Design review of the part built by this model. Coordinates are the model's own, in mm. Give positions to 0.01 mm unless a question says otherwise; leave off trailing zeros. Write each loop counter-clockwise with the first axis right and the second up, starting at its lowest first coordinate (ties: lowest second). Pieces come first, ordered by that corner, then holes. Notation, with made-up numbers: (1, -30.5) -> (25, -30.5) arc R36 ccw to (25, 8.5) -> close; hole circle Ø2 at (-30.5, -14.5). An arc over 180 degrees is marked (long way). Answer as a JSON object with one key per item and string values.
```python
from build123d import *

# Parameters (mm, degrees)
BOSS_EXTRU_1_DEPTH           = 1.6
BOSS_EXTRU_2_DEPTH           = 1.6
R_P_TITION_CIRCULAIRE1_COUNT = 24


with BuildPart() as part:
    # Esquisse1 → Boss.-Extru.1 (new body)
    with BuildSketch(Plane(origin=(0, 0, 0), x_dir=(1, 0, 0), z_dir=(0, 1, 0))):
        with BuildLine():
            ThreePointArc((12.993844697, -0.4), (-13, 0), (12.993844697, 0.4))
            Line((12.993844697, 0.4), (13.994284548, 0.4))
            ThreePointArc((13.994284548, 0.4), (-14, 0), (13.994284548, -0.4))
            Line((13.994284548, -0.4), (12.993844697, -0.4))
        make_face()
        with BuildLine():
            Line((13.994284548, 0.4), (12.993844697, 0.4))
            ThreePointArc((12.993844697, 0.4), (12.998461083, 0.200023678), (13, 0))
            ThreePointArc((13, 0), (12.998461083, -0.200023678), (12.993844697, -0.4))
            Line((12.993844697, -0.4), (13.994284548, -0.4))
            ThreePointArc((13.994284548, -0.4), (13.998571064, -0.200020415), (14, 0))
            ThreePointArc((14, 0), (13.998571064, 0.200020415), (13.994284548, 0.4))
        make_face()
    extrude(amount=BOSS_EXTRU_1_DEPTH)

    # Esquisse1<3> → Boss.-Extru.2 (add)
    with BuildSketch(Plane(origin=(0, 0, 0), x_dir=(1, 0, 0), z_dir=(0, 1, 0))):
        with BuildLine():
            Line((15.8, 0.4), (13.994284548, 0.4))
            ThreePointArc((13.994284548, 0.4), (13.998571064, 0.200020415), (14, 0))
            ThreePointArc((14, 0), (13.998571064, -0.200020415), (13.994284548, -0.4))
            Line((13.994284548, -0.4), (15.8, -0.4))
            Line((15.8, -0.4), (15.8, 0.4))
        make_face()
    boss_extru_2 = extrude(amount=BOSS_EXTRU_2_DEPTH)

    # Répétition circulaire1: Boss.-Extru.2 ×24 about axis
    r_p_tition_circulaire1_axis = Axis((0, 0, 0), (0, 1, 0))
    for i in range(1, R_P_TITION_CIRCULAIRE1_COUNT):
        add(boss_extru_2.rotate(r_p_tition_circulaire1_axis, i * 360 / R_P_TITION_CIRCULAIRE1_COUNT))


solid = part.part
```
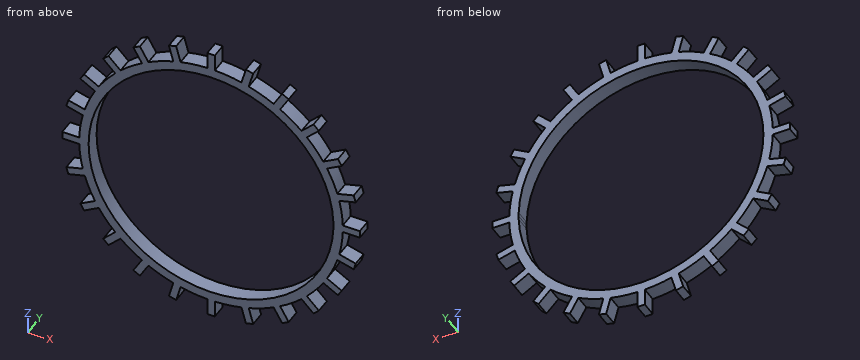
(1) Clearance check with flat-ended pins moving along their axes: pin 1 (0.5 mm diameter, centred on y = 0.5, z = 15, fed in from -X); pin 2 (0.5 mm diameter, centred on x = 15, y = 1, fed in from +Z); pin 3 (0.5 mm diameter, centred on x = 15, y = 0.5, fed in from -Z). State where each tip first meets the part, or that it passes through.
Here are the results:
{"pin 1": "stops at x = -4.48", "pin 2": "stops at z = 4.48", "pin 3": "stops at z = -4.48"}
(2) For line 1 along Z through (x, y) = (0, 1.05); line 2 along X through (y, z) = (0.95, 14.5); line 3 along Z through (x, y) = (-10.5, 1.45), list the stretches that pass through material, from the lowest coordinate up.
Here are the results:
{"line 1": "z = -15.8 to -13, 13 to 15.8", "line 2": "x = -4.3 to -3.47, -0.4 to 0.4, 3.47 to 4.3", "line 3": "z = -11.07 to -9.93, -9.26 to -7.66, 7.66 to 9.26, 9.93 to 11.07"}
(3) We need section A-A, the plane x = 0. State the section outline as (y, z) points.
Here are the results:
{"outline": "(0, -15.8) -> (1.6, -15.8) -> (1.6, -13) -> (0, -13) -> close; (0, 13) -> (1.6, 13) -> (1.6, 15.8) -> (0, 15.8) -> close"}
(4) We need section B-B, the plane z = -2. State the section outline as (x, y) points, then the cut area to 3 significant figures.
Here are the results:
{"outline": "(-13.86, 0) -> (-12.85, 0) -> (-12.85, 1.6) -> (-13.86, 1.6) -> close; (12.85, 0) -> (13.86, 0) -> (13.86, 1.6) -> (12.85, 1.6) -> close", "area": "3.24 mm²"}
